```python
from build123d import *

# Parameters (mm, degrees)
F0_R          = 17.45542
F1_DEPTH      = 46.99
F2_W          = 92.362424
F2_H          = 7.579895
F3_DEPTH      = 17.272
F3_DEPTH_BACK = 15.494
F5_DEPTH      = 5.842
F5_DEPTH_BACK = 5.334


with BuildPart() as f1:
    # F0 (on Top) → F1 (new body)
    with BuildSketch(Plane.XY):
        with BuildLine():
            ThreePointArc((68.056495, 0), (53.064586, 24.225442), (24.695165, 21.616736))
            ThreePointArc((24.695165, 21.616736), (13.918667, 0), (24.695165, -21.616736))
            ThreePointArc((24.695165, -21.616736), (53.064586, -24.225442), (68.056495, 0))
        make_face()
        with Locations((40.987581, 0)):
            Circle(F0_R, mode=Mode.SUBTRACT)
    extrude(amount=F1_DEPTH)

    # F2 (on Front) → F3 (join, two sides)
    with BuildSketch(Plane.XZ) as f3_sk:
        with Locations((-25.326473, 3.789947)):
            Rectangle(F2_W, F2_H)
    extrude(amount=F3_DEPTH)
    extrude(f3_sk.sketch, amount=-F3_DEPTH_BACK)

    # F4 (on Front) → F5 (join, two sides)
    with BuildSketch(Plane.XZ) as f5_sk:
        Polygon((14.428656, 46.435788), (-58.51711, 7.69881), (14.428656, 7.69881), align=None)
    extrude(amount=F5_DEPTH)
    extrude(f5_sk.sketch, amount=-F5_DEPTH_BACK)


solid = f1.part
```
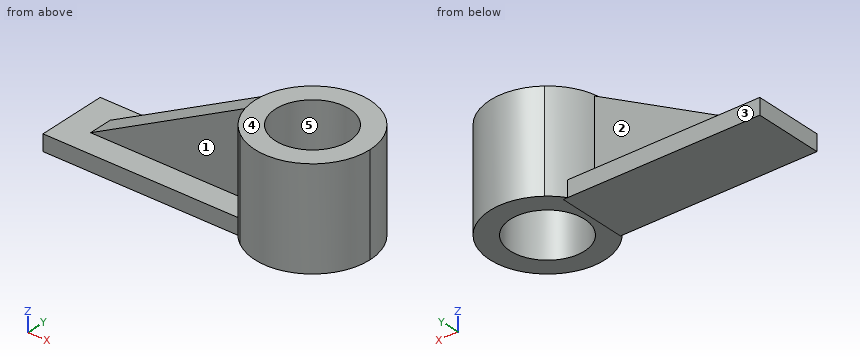
The model under review builds one solid part; all positions refer to its coordinate system, in mm. Face numbers are marked on the shaded views. A direction names the side the tool comes from. Round coordinates to 2 decimals unless told otherwise and drop trailing zeros. Write each loop counter-clockwise with the first axis right and the second up, starting at its lowest first coordinate (ties: lowest second). Pieces come first, ordered by that corner, then holes.
(1) We need section B-B on y = -12. Give the boundary of the cut face in (x, z), and give its area (3 significant figures).
(2) Mouldability with a two-part tool opening along Y and no side actions: class the marked faces 3, 4 and 5 as +Y half, -Y half, draft (parallel to the pull), parting line (faces both ways), or undercut.
(3) We need section C-C on x = -17.5. Give the boundary of the cut face in (y, z).
(4) We need section D-D on x = 17. Give the boundary of the cut face in (y, z).
(5) Wall thickness on L1, parallel to Z at x = 11, y = -9; L2, parallel to X at y = 8, z = 41; L3, parallel to Y at x = -16.5, z = 26: over which ranges is each line inside the solid? List them lowest first.
(6) We need section A-A on z = 4.5. Give the boundary of the cut face in (x, y), and give its area (3 significant figures).
(7) Machinability: for the marked faces 1 and 2, which of the approach directions +Z, -Z, +X, -X, +Y, -Y give a long, thin tool a straight path to every point of the face, cutting with its end or side? Answer none if there is none.
(8) Insertion check: pin 1 (8 mm diameter, centred on y = -6.5, z = 33, fed in from +X); pin 2 (4 mm diameter, centred on x = 12, z = 34, fed in from +Y); pin 3 (16.5 mm diameter, centred on x = -6, y = -1.5, fed in from +Z). Each pin has a flat end and moves straight along its axis. Give the tip position at first contact, or say it passes through.
Findings below:
1. outline: (-71.51, 0) - (28.31, 0) - (28.31, 46.99) - (16.72, 46.99) - (16.72, 7.58) - (-71.51, 7.58) - close; (53.66, 0) - (65.25, 0) - (65.25, 46.99) - (53.66, 46.99) - close
1. area: 1,760 mm2
2. face 3: +Y half
2. face 4: draft
2. face 5: undercut
3. outline: (-17.27, 0) - (15.49, 0) - (15.49, 7.58) - (-17.27, 7.58) - close; (-5.84, 7.7) - (5.33, 7.7) - (5.33, 29.48) - (-5.84, 29.48) - close
4. outline: (-17.27, 0) - (15.49, 0) - (15.49, 7.58) - (12.54, 7.58) - (12.54, 46.99) - (-12.54, 46.99) - (-12.54, 7.58) - (-17.27, 7.58) - close
5. L1: z = 0 to 7.58
5. L2: x = 15.13 to 25.47, 56.5 to 66.85
5. L3: y = -5.84 to 5.33
6. outline: (-71.51, -17.27) - (20.15, -17.27) arc R27.07 ccw (long way) to (18.79, 15.49) - (-71.51, 15.49) - close; hole circle Ø34.91 at (40.99, 0)
6. area: 4,200 mm2
7. face 1: +Z, -X, -Y
7. face 2: +Z, -X, +Y
8. pin 1: stops at x = 67.94
8. pin 2: stops at y = 5.33
8. pin 3: stops at z = 39.97
